```python
from build123d import *

# Parameters (mm, degrees)
F1_DEPTH = 203.2
F2_R     = 1.5875
F3_DEPTH = 25.4
F4_R     = 1.5875
F5_DEPTH = 25.4


with BuildPart() as f1:
    # F0 (on Top) → F1 (new body)
    with BuildSketch(Plane.XY):
        with BuildLine():
            Line((-25.4, -38.1), (28.575, -38.1))
            ThreePointArc((28.575, -38.1), (35.310192, -35.310192), (38.1, -28.575))
            Line((38.1, -28.575), (38.1, 25.4))
            ThreePointArc((38.1, 25.4), (34.380256, 34.380256), (25.4, 38.1))
            Line((25.4, 38.1), (-25.4, 38.1))
            ThreePointArc((-25.4, 38.1), (-34.380256, 34.380256), (-38.1, 25.4))
            Line((-38.1, 25.4), (-38.1, -25.4))
            ThreePointArc((-38.1, -25.4), (-34.380256, -34.380256), (-25.4, -38.1))
        make_face()
        with BuildLine():
            ThreePointArc((28.575, -22.225), (26.715128, -26.715128), (22.225, -28.575))
            Line((22.225, -28.575), (-22.225, -28.575))
            ThreePointArc((-22.225, -28.575), (-26.715128, -26.715128), (-28.575, -22.225))
            Line((-28.575, -22.225), (-28.575, 22.225))
            ThreePointArc((-28.575, 22.225), (-26.715128, 26.715128), (-22.225, 28.575))
            Line((-22.225, 28.575), (22.225, 28.575))
            ThreePointArc((22.225, 28.575), (26.715128, 26.715128), (28.575, 22.225))
            Line((28.575, 22.225), (28.575, -22.225))
        make_face(mode=Mode.SUBTRACT)
    extrude(amount=F1_DEPTH)

    # F2 (on face) → F3 (cut)
    with BuildSketch(Plane.XY.offset(203.2)):
        with Locations((-33.3375, 19.05)):
            Circle(F2_R)
        with Locations((-33.3375, -19.05)):
            Circle(F2_R)
        with Locations((33.3375, -19.05)):
            Circle(F2_R)
        with Locations((33.3375, 19.05)):
            Circle(F2_R)
    extrude(amount=-F3_DEPTH, mode=Mode.SUBTRACT)

    # F4 (on face) → F5 (cut)
    with BuildSketch(Plane(origin=(0, 0, 0), x_dir=(1, 0, 0), z_dir=(0, 0, -1))):
        with Locations((-33.3375, 19.05)):
            Circle(F4_R)
        with Locations((-33.3375, -19.05)):
            Circle(F4_R)
        with Locations((33.3375, 19.05)):
            Circle(F4_R)
        with Locations((33.3375, -19.05)):
            Circle(F4_R)
    extrude(amount=-F5_DEPTH, mode=Mode.SUBTRACT)


solid = f1.part
```
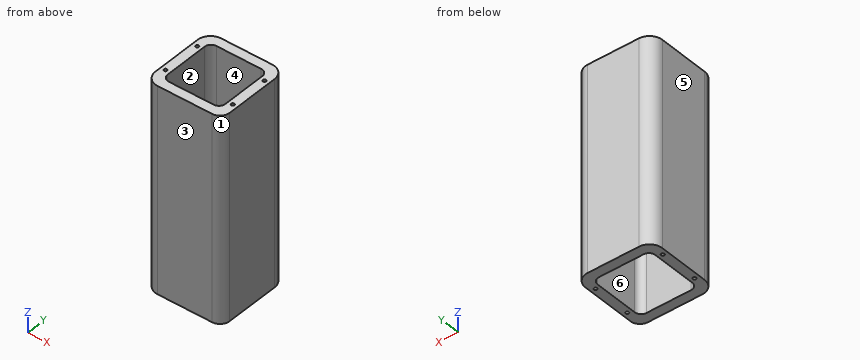
Check sheet for the modelled part. Datum: model origin and axes. Units: mm. Face numbers are marked on the shaded views. A direction names the side the tool comes from. Round coordinates to 2 decimals unless told otherwise and drop trailing zeros. Order: outer loops, then holes, each group sorted by start corner. A loop starts at its lowest first (then second) coordinate and runs counter-clockwise, first axis right, second up. Notation, with made-up numbers: (31.5, 66.25) - (82.5, 66.25) arc R23 cw to (82.5, 99.25) - close; hole circle Ø2 at (-37.5, 15.5). An arc over 180 degrees is marked (long way). Answer as CSV lines item,"result". Start each with the question number.
1) Tool access check on the marked faces 5 and 6. Record the directions out of +Z, -Z, +X, -X, +Y, -Y that give a thin tool (end or side, any length) a straight path to the whole face; none if there is none.
2) Section check A-A (x = -1). Record the cut outline in (y, z) (3 decimals), then the cut area to 3 significant figures.
3) Depth check by flat-ended pin: pin 1 (5 mm diameter, centred on x = 29.5, z = 94.5, fed in from +Y); pin 2 (1.9 mm diameter, centred on x = -33.34, y = -19.05, fed in from -Z); pin 3 (3 mm diameter, centred on x = -33.34, y = 19.05, fed in from +Z). Enter the tip coordinate at first touch or a pass-through.
4) Section check C-C (z = 37.5). Record the cut outline in (x, y) (3 decimals), then the cut area to 3 significant figures.
5) Draft check along X on the marked faces 1, 2, 3 and 4. Enter one of: +X half, -X half, draft (parallel to the pull), parting line (faces both ways), or undercut.
6) Scan lines: probe 1 along X at (y, z) = (19.05, 14.5) (3 decimals); probe 2 along X at (y, z) = (-12, 65.5) (3 decimals). Record each from-to range of solid material in increasing order.
Determined:
1,face 5,"+Z, -Z, -X, +Y, -Y"
1,face 6,"+Z, -Z"
2,outline,"(-38.1, 0) - (-28.575, 0) - (-28.575, 203.2) - (-38.1, 203.2) - close; (28.575, 0) - (38.1, 0) - (38.1, 203.2) - (28.575, 203.2) - close"
2,area,"3,870 mm^2"
3,pin 1,"y = 38"
3,pin 2,"z = 25.4"
3,pin 3,"z = 177.8"
4,outline,"(-38.1, -25.4) arc R12.7 ccw to (-25.4, -38.1) - (28.575, -38.1) arc R9.525 ccw to (38.1, -28.575) - (38.1, 25.4) arc R12.7 ccw to (25.4, 38.1) - (-25.4, 38.1) arc R12.7 ccw to (-38.1, 25.4) - close; hole (-28.575, -22.225) arc R6.35 ccw to (-22.225, -28.575) - (22.225, -28.575) arc R6.35 ccw to (28.575, -22.225) - (28.575, 22.225) arc R6.35 ccw to (22.225, 28.575) - (-22.225, 28.575) arc R6.35 ccw to (-28.575, 22.225) - close"
4,area,"2,450 mm^2"
5,face 1,"+X half"
5,face 2,"undercut"
5,face 3,"draft"
5,face 4,"undercut"
6,probe 1,"-38.1 to -34.925, -31.75 to -28.575, 28.575 to 31.75, 34.925 to 38.1"
6,probe 2,"-38.1 to -28.575, 28.575 to 38.1"
